from build123d import *

# Parameters (mm, degrees)
BOSS_EXTRUDE1_DEPTH = 20
SKETCH2_R           = 2
CUT_EXTRUDE1_DEPTH  = 20
FILLET1_R           = 2
FILLET2_R           = 1
SKETCH3_R           = 3
BOSS_EXTRUDE2_DEPTH = 5


with BuildPart() as part:
    # Sketch1 → Boss-Extrude1 (new body)
    with BuildSketch(Plane.XY):
        with BuildLine():
            Line((20, 14), (27, 14))
            Line((27, 14), (27, 17))
            Line((27, 17), (20, 17))
            Line((20, 17), (20, 25))
            ThreePointArc((20, 25), (19.707106781, 25.707106781), (19, 26))
            Line((19, 26), (-19, 26))
            ThreePointArc((-19, 26), (-19.707106781, 25.707106781), (-20, 25))
            Line((-20, 25), (-20, 17))
            Line((-20, 17), (-27, 17))
            Line((-27, 17), (-27, 14))
            Line((-27, 14), (-20, 14))
            Line((-20, 14), (-20, -14))
            Line((-20, -14), (20, -14))
            Line((20, -14), (20, 14))
        make_face()
    extrude(amount=BOSS_EXTRUDE1_DEPTH)

    # Sketch2 → Cut-Extrude1 (cut)
    with BuildSketch(Plane(origin=(0, 17, 0), x_dir=(1, 0, 0), z_dir=(0, 1, 0))):
        with Locations(Location((-24.5, -5, 0), (0, 0, 270))):
            Circle(SKETCH2_R)
        with Locations(Location((-24.5, -15, 0), (0, 0, 270))):
            Circle(SKETCH2_R)
    cut_extrude1 = extrude(amount=-CUT_EXTRUDE1_DEPTH, mode=Mode.SUBTRACT)

    # Mirror1: Cut-Extrude1 across plane
    add(cut_extrude1.mirror(Plane(origin=(0, 0, 0), x_dir=(0, 0, 1), z_dir=(1, 0, 0))), mode=Mode.SUBTRACT)

    # Fillet1
    fillet1_edges = [part.edges().sort_by_distance(p)[0] for p in [
        (27, 15.5, 20),
        (-27, 15.5, 0),
        (27, 15.5, 0),
        (-27, 15.5, 20),
    ]]
    fillet(fillet1_edges, radius=FILLET1_R)

    # Fillet2
    fillet2_edges = [part.edges().sort_by_distance(p)[0] for p in [
        (-20, 0, 0),
        (-20, 21, 0),
        (-19.707106781, 25.707106781, 0),
        (0, 26, 0),
        (19.707106781, 25.707106781, 0),
        (20, 21, 0),
        (20, 0, 0),
        (20, 21, 20),
        (19.707106781, 25.707106781, 20),
        (0, 26, 20),
        (-19.707106781, 25.707106781, 20),
        (-20, 21, 20),
        (20, 0, 20),
        (-20, 0, 20),
    ]]
    fillet(fillet2_edges, radius=FILLET2_R)

    # Sketch3 → Boss-Extrude2 (add)
    with BuildSketch(Plane(origin=(0, 26, 0), x_dir=(1, 0, 0), z_dir=(0, 1, 0))):
        with Locations(Location((11, -10, 0), (0, 0, 270))):
            Circle(SKETCH3_R)
    extrude(amount=BOSS_EXTRUDE2_DEPTH)


solid = part.part
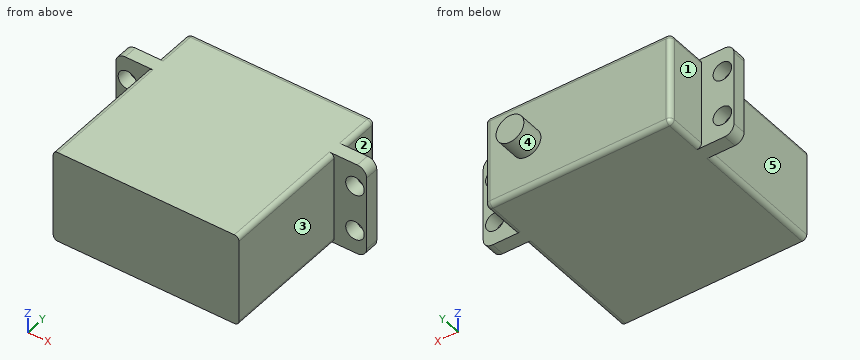
Can you work these out from the model? Positions are in its coordinate system, mm. Face numbers are marked on the shaded views. A direction names the side the tool comes from. Give positions to 0.01 mm unless a question says otherwise; leave off trailing zeros. Order: outer loops, then holes, each group sorted by start corner. A loop starts at its lowest first (then second) coordinate and runs counter-clockwise, first axis right, second up. Notation, with made-up numbers: M 42.25,56 L 50.25,56 A23 cw 50.25,81 Z; hole C 59,21 d7. An arc over 180 degrees is marked long. Use a Markdown table: item, result. Add a question column.
Item 1: Will these pins go through, and if not, where does the flat tip stop? pin 1 (2 mm diameter, centred on y = 10.5, z = 11.5, fed in from -X); pin 2 (6.5 mm diameter, centred on x = -22.5, z = 13.5, fed in from +Y); pin 3 (8 mm diameter, centred on y = -4, z = 4.5, fed in from +X).
Item 2: Suppose I cut it at C-C (x = 11). List the corners of the cut face in (y, z) for me.
Item 3: For the marked faces 1, 2, 3, 4 and 5, which set-ups out of +Z, -Z, +X, -X, +Y, -Y let a thin tool reach every point of the face, with its end or its side?
Item 4: Suppose I cut it at B-B (y = 19.5). List the corners of the cut face in (x, z) for me, then the cut area to 3 significant figures.
Item 5: If I drill on L1, parallel to Z at x = 24.5, y = 15.3; L2, parallel to X at y = 15.8, z = 15; L3, parallel to Z at x = -24, y = 15, over which ranges is the centre line in solid material (lowest first)? Write a range as [from, to].
Item 6: Suppose I cut it at A-A (z = 15). List the corners of the cut face in (x, y) for me, then the cut area to 3 significant figures.
Answer sheet:
| question | item | result |
|---|---|---|
| 1 | pin 1 | stops at x = -20 |
| 1 | pin 2 | stops at y = 25.97 |
| 1 | pin 3 | stops at x = 20 |
| 2 | outline | M -14,0 L 25,0 A1 ccw 26,1 L 26,7 L 31,7 L 31,13 L 26,13 L 26,19 A1 ccw 25,20 L -14,20 Z |
| 3 | face 1 | +Z, -Z, -X, +Y |
| 3 | face 2 | +Z, -Z, +X, +Y |
| 3 | face 3 | +Z, -Z, +X, -Y |
| 3 | face 4 | +Y |
| 3 | face 5 | +Z, -Z, -X, -Y |
| 4 | outline | M -20,1 A1 ccw -19,0 L 19,0 A1 ccw 20,1 L 20,19 A1 ccw 19,20 L -19,20 A1 ccw -20,19 Z |
| 4 | area | 799 mm² |
| 5 | L1 | z = [0, 3], [7, 13], [17, 20] |
| 5 | L2 | x = [-27, -26.5], [-22.5, 22.5], [26.5, 27] |
| 5 | L3 | z = [0, 3.06], [6.94, 13.06], [16.94, 20] |
| 6 | outline | M -27,14 L -26.5,14 L -26.5,17 L -27,17 Z; M -22.5,14 L -20,14 L -20,-14 L 20,-14 L 20,14 L 22.5,14 L 22.5,17 L 20,17 L 20,25 A1 ccw 19,26 L -19,26 A1 ccw -20,25 L -20,17 L -22.5,17 Z; M 26.5,14 L 27,14 L 27,17 L 26.5,17 Z |
| 6 | area | 1,620 mm² |
